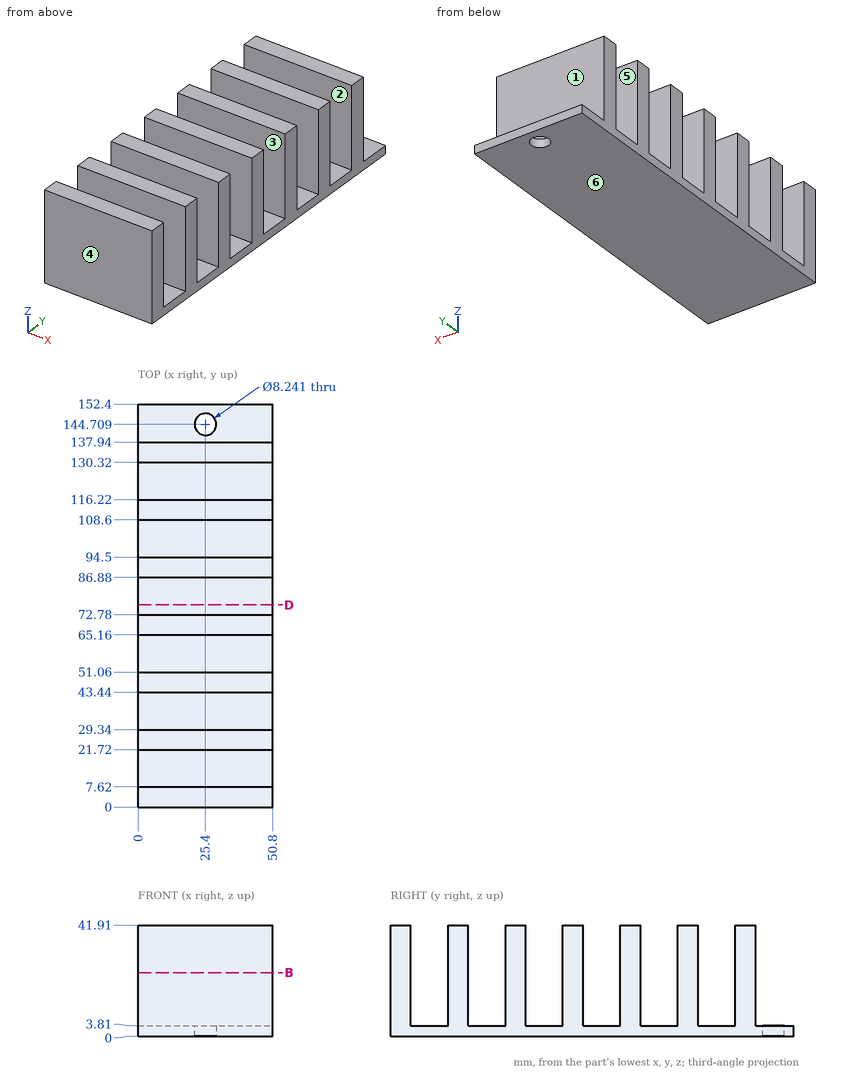
Can you work these out from the drawing? Everything is in mm from the part's minimum corner. A direction names the side the tool comes from. Give positions to 0.01 mm unless a question says otherwise; leave off trailing zeros. Order: outer loops, then holes, each group sorted by start corner. A loop starts at its lowest first (then second) coordinate and runs counter-clockwise, first axis right, second up. Notation, with made-up numbers: M 66,-22 L 106,-22 A34 ccw 106,12 Z; hole C 10.25,82.25 d11. An arc over 180 degrees is marked long. One line per item, written item: value.
Item 1: For the marked faces 5 and 6, which set-ups out of +Z, -Z, +X, -X, +Y, -Y let a thin tool reach every point of the face, with its end or its side?
Verdict:
face 5: +Z, +X, -X
face 6: -Z, +X, -X, +Y, -Y
Item 2: If we section it at D-D on y = 76.5: Write out the boundary of the cut face in (x, z).
Verdict:
outline: M 0,0 L 50.8,0 L 50.8,3.81 L 0,3.81 Z
Item 3: For pin 1 (1 mm diameter, centred on x = 6, z = 12.5, fed in from +Y); pin 2 (7 mm diameter, centred on x = 13, y = 12, fed in from +Z), each with a flat end and sliding along its axis, tell me the tip position at first contact or that it passes through.
Verdict:
pin 1: y = 137.94
pin 2: z = 3.81
Item 4: Please list where these lines run through material, in increasing order: line 1 (Y direction, x = 25.4, z = 1.6); line 2 (Z direction, x = 17, y = 139.5).
Verdict:
line 1: 0 to 140.59, 148.83 to 152.4
line 2: 0 to 3.81
Item 5: If we mould it in two halves opening along Y, with no side actions, what happens to the marked faces 1, 2, 3 and 4? For each: pulls with the +Y half, pulls with the -Y half, needs draft (parallel to the pull), parting line crosses it, or undercut.
Verdict:
face 1: pulls with the +Y half
face 2: undercut
face 3: undercut
face 4: pulls with the -Y half
Item 6: If we section it at B-B on z = 24: Write out the boundary of the cut face in (x, y).
Verdict:
outline: M 0,0 L 50.8,0 L 50.8,7.62 L 0,7.62 Z; M 0,21.72 L 50.8,21.72 L 50.8,29.34 L 0,29.34 Z; M 0,43.44 L 50.8,43.44 L 50.8,51.06 L 0,51.06 Z; M 0,65.16 L 50.8,65.16 L 50.8,72.78 L 0,72.78 Z; M 0,86.88 L 50.8,86.88 L 50.8,94.5 L 0,94.5 Z; M 0,108.6 L 50.8,108.6 L 50.8,116.22 L 0,116.22 Z; M 0,130.32 L 50.8,130.32 L 50.8,137.94 L 0,137.94 Z
